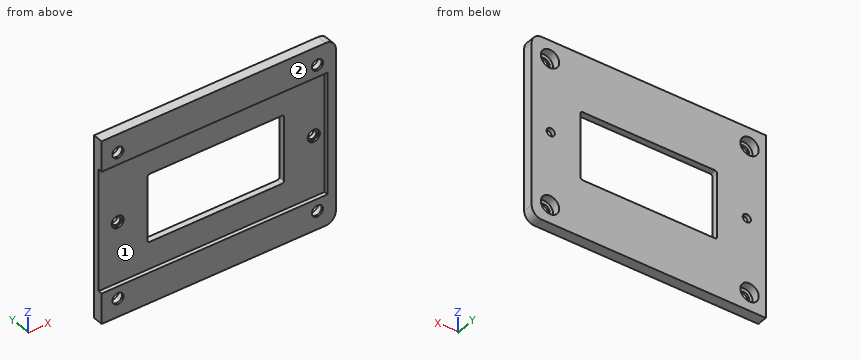
from build123d import *

# Parameters (mm, degrees)
SKETCH1_W                      = 115
SKETCH1_H                      = 90
SKETCH1_W_2                    = 67
SKETCH1_H_2                    = 33.5
BOSS_EXTRUDE1_DEPTH            = 5
FILLET1_R                      = 5
FILLET2_R                      = 1
CBORE_FOR_M5_SHCS1_D           = 5.5
CBORE_FOR_M5_SHCS1_CBORE_D     = 9
CBORE_FOR_M5_SHCS1_CBORE_DEPTH = 4
SKETCH5_W                      = 111
SKETCH5_H                      = 60
CUT_EXTRUDE1_DEPTH             = 2
CBORE_FOR_M5_SHCS2_D           = 4
CBORE_FOR_M5_SHCS2_CBORE_D     = 6
CBORE_FOR_M5_SHCS2_CBORE_DEPTH = 1


with BuildPart() as part:
    # Sketch1 → Boss-Extrude1 (new body)
    with BuildSketch(Plane(origin=(0, 0, 0), x_dir=(1, 0, 0), z_dir=(0, 1, 0))):
        Rectangle(SKETCH1_W, SKETCH1_H)
        Rectangle(SKETCH1_W_2, SKETCH1_H_2, mode=Mode.SUBTRACT)
    extrude(amount=BOSS_EXTRUDE1_DEPTH)

    # Fillet1
    fillet1_edges = [part.edges().sort_by_distance(p)[0] for p in [
        (57.5, 2.5, -45),
        (57.5, 2.5, 45),
    ]]
    fillet(fillet1_edges, radius=FILLET1_R)

    # Fillet2
    fillet2_edges = [part.edges().sort_by_distance(p)[0] for p in [
        (-33.5, 2.5, 16.75),
        (33.5, 2.5, 16.75),
        (33.5, 2.5, -16.75),
        (-33.5, 2.5, -16.75),
    ]]
    fillet(fillet2_edges, radius=FILLET2_R)

    # CBORE for M5 SHCS1 (through all)
    with Locations(Plane(origin=(0, 5, 0), x_dir=(1, 0, 0), z_dir=(0, 1, 0))):
        with Locations((-49.5, 36), (-49.5, -36), (48.5, -36), (48.5, 36)):
            CounterBoreHole(CBORE_FOR_M5_SHCS1_D / 2, CBORE_FOR_M5_SHCS1_CBORE_D / 2, CBORE_FOR_M5_SHCS1_CBORE_DEPTH)

    # Sketch5 → Cut-Extrude1 (cut)
    with BuildSketch(Plane.XZ):
        with Locations((-2, 0)):
            Rectangle(SKETCH5_W, SKETCH5_H)
    extrude(amount=-CUT_EXTRUDE1_DEPTH, mode=Mode.SUBTRACT)

    # CBORE for M5 SHCS2 (through all)
    with Locations(Plane(origin=(0, 2, 0), x_dir=(-1, 0, 0), z_dir=(0, -1, 0))):
        with Locations((48.15, 0), (-48.15, 0)):
            CounterBoreHole(CBORE_FOR_M5_SHCS2_D / 2, CBORE_FOR_M5_SHCS2_CBORE_D / 2, CBORE_FOR_M5_SHCS2_CBORE_DEPTH)


solid = part.part
Read the model definition and answer for the solid it produces. Units are mm, in the model's axes. Face numbers are marked on the shaded views. Round coordinates to 2 decimals unless told otherwise and drop trailing zeros. Order: outer loops, then holes, each group sorted by start corner. A loop starts at its lowest first (then second) coordinate and runs counter-clockwise, first axis right, second up. Notation, with made-up numbers: (-23.75, 12.25) - (7.25, 12.25) arc R8 ccw to (7.25, 23.25) - close; hole circle Ø8 at (-30.5, -3.5). An arc over 180 degrees is marked (long way). Use one line per item in the form item = value. Start each with the question number.
(1) Find the intervals of material crossed by line 1 along X through (y, z) = (2.9, 36); line 2 along Z through (x, y) = (48.5, 0.3); line 3 along X through (y, z) = (0.65, -36), in increasing order. Write a range as from..to.
(2) The part is cut by section B-B (z = 0). Give the vertices of the cut face in (x, y), then the cut area to 3 significant figures.
(3) Flat-ended cylindrical pins translate along their axes: pin 1 Ø7 at (x, z) = (-49.5, 36) entering from +Y; pin 2 Ø5 at (x, z) = (-49, 0.5) entering from -Y; pin 3 Ø1.6 at (y, z) = (1, -10.5) entering from -X. Find the tip coordinate at first contact, or state that the pin passes through.
(4) The part is cut by section C-C (z = -9). Give the vertices of the cut face in (x, y), then the cut area to 3 significant figures.
(5) The part is cut by section D-D (x = 48.5). Count the separate pieces of the cut face and the enclosed holes in it, then the cut area to 3 significant figures.
(6) The part is cut by section A-A (x = 25.5). Give the vertices of the cut face in (y, z).
(7) Determine the mould class of the marked faces 1 and 2 for opening direction Z: +Z half, -Z half, draft (parallel to the pull), parting line (faces both ways), or undercut.
Checked values:
q1.line_1 = -57.5..-54, -45..44, 53..57.5
q1.line_2 = -45..-38.75, -33.25..-30, 30..33.25, 38.75..45
q1.line_3 = -57.5..-52.25, -46.75..45.75, 51.25..57.5
q2.outline = (-57.5, 2) - (-51.15, 2) - (-51.15, 3) - (-50.15, 3) - (-50.15, 5) - (-57.5, 5) - close; (-46.15, 3) - (-45.15, 3) - (-45.15, 2) - (-33.5, 2) - (-33.5, 5) - (-46.15, 5) - close; (33.5, 2) - (45.15, 2) - (45.15, 3) - (46.15, 3) - (46.15, 5) - (33.5, 5) - close; (50.15, 3) - (51.15, 3) - (51.15, 2) - (53.5, 2) - (53.5, 0) - (57.5, 0) - (57.5, 5) - (50.15, 5) - close
q2.area = 124 mm^2
q3.pin_1 = 1
q3.pin_2 = 2
q3.pin_3 = 53.5
q4.outline = (-57.5, 2) - (-33.5, 2) - (-33.5, 5) - (-57.5, 5) - close; (33.5, 2) - (53.5, 2) - (53.5, 0) - (57.5, 0) - (57.5, 5) - (33.5, 5) - close
q4.area = 152 mm^2
q5.separate_pieces = 4
q5.enclosed_holes = 0
q5.area = 233 mm^2
q6.outline = (0, -45) - (5, -45) - (5, -16.75) - (2, -16.75) - (2, -30) - (0, -30) - close; (0, 30) - (2, 30) - (2, 16.75) - (5, 16.75) - (5, 45) - (0, 45) - close
q7.face_1 = undercut
q7.face_2 = draft
